from build123d import *

# Parameters (mm, degrees)
ESBO_O1_R                = 1.25
ESBO_O1_R_2              = 1.6
ESBO_O1_R_3              = 7
RESSALTO_EXTRUS_O1_DEPTH = 4.5
ESBO_O2_W                = 9.082800448
ESBO_O2_H                = 32.5
CORTE_EXTRUS_O1_DEPTH    = 5.5
FILETE1_R                = 2


with BuildPart() as part:
    # Esboço1 → Ressalto-extrusão1 (new body)
    with BuildSketch(Plane(origin=(0, 0, -4.5), x_dir=(-1, 0, 0), z_dir=(0, 0, -1))):
        with BuildLine():
            Line((-10.853553391, -14.896446609), (-9.646446609, -16.103553391))
            ThreePointArc((-9.646446609, -16.103553391), (-9.484234935, -16.211939766), (-9.292893219, -16.25))
            Line((-9.292893219, -16.25), (-2.1, -16.25))
            ThreePointArc((-2.1, -16.25), (-1.746446609, -16.103553391), (-1.6, -15.75))
            Line((-1.6, -15.75), (-1.6, -13.856406461))
            ThreePointArc((-1.6, -13.856406461), (0, -12.256406461), (1.6, -13.856406461))
            Line((1.6, -13.856406461), (1.6, -15.75))
            ThreePointArc((1.6, -15.75), (1.746446609, -16.103553391), (2.1, -16.25))
            Line((2.1, -16.25), (9.292893219, -16.25))
            ThreePointArc((9.292893219, -16.25), (9.484234935, -16.211939766), (9.646446609, -16.103553391))
            Line((9.646446609, -16.103553391), (10.853553391, -14.896446609))
            ThreePointArc((10.853553391, -14.896446609), (10.961939766, -14.734234935), (11, -14.542893219))
            Line((11, -14.542893219), (11, 14.542893219))
            ThreePointArc((11, 14.542893219), (10.961939766, 14.734234935), (10.853553391, 14.896446609))
            Line((10.853553391, 14.896446609), (9.646446609, 16.103553391))
            ThreePointArc((9.646446609, 16.103553391), (9.484234935, 16.211939766), (9.292893219, 16.25))
            Line((9.292893219, 16.25), (2.1, 16.25))
            ThreePointArc((2.1, 16.25), (1.746446609, 16.103553391), (1.6, 15.75))
            Line((1.6, 15.75), (1.6, 13.856406461))
            ThreePointArc((1.6, 13.856406461), (0, 12.256406461), (-1.6, 13.856406461))
            Line((-1.6, 13.856406461), (-1.6, 15.75))
            ThreePointArc((-1.6, 15.75), (-1.746446609, 16.103553391), (-2.1, 16.25))
            Line((-2.1, 16.25), (-9.292893219, 16.25))
            ThreePointArc((-9.292893219, 16.25), (-9.484234935, 16.211939766), (-9.646446609, 16.103553391))
            Line((-9.646446609, 16.103553391), (-10.853553391, 14.896446609))
            ThreePointArc((-10.853553391, 14.896446609), (-10.961939766, 14.734234935), (-11, 14.542893219))
            Line((-11, 14.542893219), (-11, -14.542893219))
            ThreePointArc((-11, -14.542893219), (-10.961939766, -14.734234935), (-10.853553391, -14.896446609))
        make_face()
        with Locations((-8, -10)):
            Circle(ESBO_O1_R, mode=Mode.SUBTRACT)
        with Locations((8, -10)):
            Circle(ESBO_O1_R, mode=Mode.SUBTRACT)
        with Locations((8, 10)):
            Circle(ESBO_O1_R, mode=Mode.SUBTRACT)
        with Locations((-8, 10)):
            Circle(ESBO_O1_R, mode=Mode.SUBTRACT)
        with Locations((-8, -13.85640646)):
            Circle(ESBO_O1_R_2, mode=Mode.SUBTRACT)
        with Locations((8, -13.85640646)):
            Circle(ESBO_O1_R_2, mode=Mode.SUBTRACT)
        with Locations((8, 13.85640646)):
            Circle(ESBO_O1_R_2, mode=Mode.SUBTRACT)
        with Locations((-8, 13.85640646)):
            Circle(ESBO_O1_R_2, mode=Mode.SUBTRACT)
        Circle(ESBO_O1_R_3, mode=Mode.SUBTRACT)
    extrude(amount=-RESSALTO_EXTRUS_O1_DEPTH)

    # Esboço2 → Corte-extrusão1 (cut, through all)
    with BuildSketch(Plane.XY):
        with Locations((-10.842301115, 0)):
            Rectangle(ESBO_O2_W, ESBO_O2_H)
    extrude(amount=-CORTE_EXTRUS_O1_DEPTH, mode=Mode.SUBTRACT)

    # Filete1
    filete1_edges = [part.edges().sort_by_distance(p)[0] for p in [
        (-6.300900891, 16.25, -2.25),
        (-6.300900891, -16.25, -2.25),
    ]]
    fillet(filete1_edges, radius=FILETE1_R)


solid = part.part
Read the model definition and answer for the solid it produces. Units are mm, in the model's axes. A direction names the side the tool comes from. Coordinates: 2 decimals unless noted, no trailing zeros. Order: outer loops, then holes, each group sorted by start corner. A loop starts at its lowest first (then second) coordinate and runs counter-clockwise, first axis right, second up. Notation, with made-up numbers: M 44,33 L 89,33 A19 cw 89,49 Z; hole C 74.25,85.5 d10. An arc over 180 degrees is marked long. Put each result on its own line as item: value. Start each with the question number.
Item 1: The mould has two halves that part along X. Classify faces 3 (the face through (8.921, 10.845, -2.282)), 4 (the face through (6, -16.25, -2)), 5 (the face through (-1.6, 15, -2)), 6 (the face through (10.24, 15.51, -2.28)): +X half, -X half, draft (parallel to the pull), parting line (faces both ways), or undercut.
Item 2: Section A-A, the plane y = 10 is taken. Determine the outline of the cut face in (x, z).
Item 3: Section B-B, the plane x = 0 is taken. Determine the outline of the cut face in (y, z), plus the area to 3 significant figures.
Item 4: Section D-D, the plane x = 8 is taken. Determine the outline of the cut face in (y, z), plus the area to 4 significant figures.
Item 5: Given pin 1 Ø0.6 at (y, z) = (15, -1.5) entering from -X, flat-ended and moving along its own axis, determine where the tip first touches the part or whether it passes through.
Item 6: Section C-C, the plane z = -0.65 is taken. Count the separate pieces of the cut face and the enclosed holes in it, plus the area to 3 significant figures.
Item 7: For faces 1 (the face through (1.6, 15, -2)), 2 (the face through (6, 16.25, -2)), determine the directions among +Z, -Z, +X, -X, +Y, -Y from which every point of the face is accessible in a straight line to the end or side of a thin tool.
Item 8: Consider probe 1 along X at (y, z) = (14, -0.15); probe 2 along Y at (x, z) = (8, -2.4); probe 3 along Y at (x, z) = (7.5, -1.1). Determine where each line is inside the solid, lowest interval first. Write a range as [from, to].
Computed:
1. face 3: undercut
1. face 4: draft
1. face 5: undercut
1. face 6: +X half
2. outline: M -6.3,-4.5 L 6.75,-4.5 L 6.75,0 L -6.3,0 Z; M 9.25,-4.5 L 11,-4.5 L 11,0 L 9.25,0 Z
3. outline: M -12.26,-4.5 L -7,-4.5 L -7,0 L -12.26,0 Z; M 7,-4.5 L 12.26,-4.5 L 12.26,0 L 7,0 Z
3. area: 47.3 mm2
4. outline: M -16.25,-4.5 L -15.46,-4.5 L -15.46,0 L -16.25,0 Z; M -12.26,-4.5 L -11.25,-4.5 L -11.25,0 L -12.26,0 Z; M -8.75,-4.5 L 8.75,-4.5 L 8.75,0 L -8.75,0 Z; M 11.25,-4.5 L 12.26,-4.5 L 12.26,0 L 11.25,0 Z; M 15.46,-4.5 L 16.25,-4.5 L 16.25,0 L 15.46,0 Z
4. area: 94.95 mm2
5. pin 1: stops at x = -6.25
6. separate pieces: 1
6. enclosed holes: 4
6. area: 358 mm2
7. face 1: +Z, -Z, +Y
7. face 2: +Z, -Z, +X, -X, +Y
8. probe 1: x = [-6.3, -1.6], [1.6, 6.41], [9.59, 11]
8. probe 2: y = [-16.25, -15.46], [-12.26, -11.25], [-8.75, 8.75], [11.25, 12.26], [15.46, 16.25]
8. probe 3: y = [-16.25, -15.38], [-12.34, -11.15], [-8.85, 8.85], [11.15, 12.34], [15.38, 16.25]
